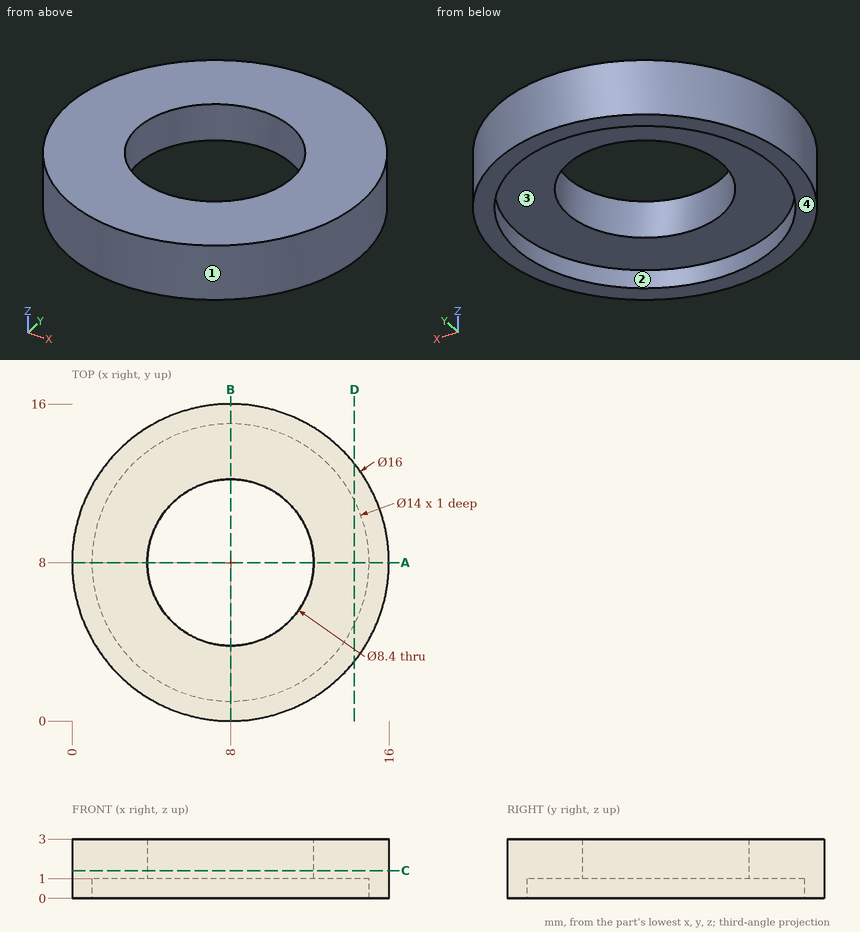
Job drawing, mm, ordinate dimensions from the low corner. One solid piece. Round coordinates to 2 decimals unless told otherwise and drop trailing zeros. Write each loop counter-clockwise with the first axis right and the second up, starting at its lowest first coordinate (ties: lowest second). Pieces come first, ordered by that corner, then holes. Notation, with made-up numbers: (-37, 1.25) -> (-12, 1.25) arc R7 ccw to (-12, 10.25) -> close; hole circle Ø9 at (84.25, 64.5). An arc over 180 degrees is marked (long way). Answer as a JSON object with one key per item and string values.
(1) Band-saw the part on C-C, the plane z = 1.4. List the corners of the cut face in (x, y).
Reported:
{"outline": "circle Ø16 at (8, 8); hole circle Ø8.4 at (8, 8)"}
(2) Band-saw the part on D-D, the plane x = 14.25. List the corners of the cut face in (y, z), then the cut area to 3 significant figures.
Reported:
{"outline": "(3.01, 0) -> (4.85, 0) -> (4.85, 1) -> (11.15, 1) -> (11.15, 0) -> (12.99, 0) -> (12.99, 3) -> (3.01, 3) -> close", "area": "23.7 mm^2"}
(3) Pin check, flat tips, straight feed: P1, Ø1, axis at x = 7.5, z = 2.5, coming from the +Y side; P2, Ø1, axis at y = 9, z = 2.5, coming from the -X side. Stop position of each tip, or through.
Reported:
{"P1": "stops at y = 16", "P2": "stops at x = 0.02"}
(4) Probe probe 1 along Y at (x, z) = (8, 1.95); probe 2 along Y at (x, z) = (8, 0.7); probe 3 along Z at (x, y) = (11.5, 10.5). List the from-to ranges inside material, lowest first. Write a range as [from, to].
Reported:
{"probe 1": "y = [0, 3.8], [12.2, 16]", "probe 2": "y = [0, 1], [15, 16]", "probe 3": "z = [1, 3]"}
(5) Band-saw the part on A-A, the plane y = 8. List the corners of the cut face in (x, z), then the cut area to 3 significant figures.
Reported:
{"outline": "(0, 0) -> (1, 0) -> (1, 1) -> (3.8, 1) -> (3.8, 3) -> (0, 3) -> close; (12.2, 1) -> (15, 1) -> (15, 0) -> (16, 0) -> (16, 3) -> (12.2, 3) -> close", "area": "17.2 mm^2"}
(6) Two-plate mould, pull along X, no slides. Class the marked faces 1, 2, 3 and 4: +X half, -X half, draft (parallel to the pull), parting line (faces both ways), or undercut.
Reported:
{"face 1": "parting line", "face 2": "undercut", "face 3": "undercut", "face 4": "draft"}
